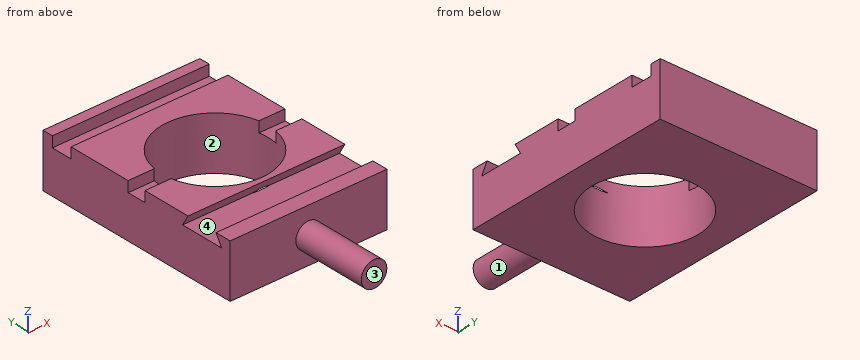
```python
from build123d import *

# Parameters (mm, degrees)
F1_W      = 73.6989242806
F1_H      = 100
F1_R      = 25
F2_DEPTH  = 100
F3_W      = 73.6989242806
F3_H      = 10
F4_DEPTH  = 5
F6_DEPTH  = 73.6989242806
F0_W      = 73.6989242806
F0_H      = 100
F7_DEPTH  = 75
F8_DEPTH  = 75
F9_R      = 6
F10_DEPTH = 35


with BuildPart() as f2:
    # F1 (on face) → F2 (new body)
    with BuildSketch(Plane.XY):
        Rectangle(F1_W, F1_H)
        Circle(F1_R, mode=Mode.SUBTRACT)
    extrude(amount=F2_DEPTH)

    # F3 (on face) → F4 (cut)
    with BuildSketch(Plane.XY.offset(100)):
        with BuildLine():
            Line((-24.5916652547, 4.5), (-36.8494621403, 4.5))
            Line((-36.8494621403, 4.5), (-36.8494621403, -4.5))
            Line((-36.8494621403, -4.5), (-24.5916652547, -4.5))
            ThreePointArc((-24.5916652547, -4.5), (-25, 0), (-24.5916652547, 4.5))
        make_face()
        with BuildLine():
            Line((36.8494621403, -4.5), (36.8494621403, 4.5))
            Line((36.8494621403, 4.5), (24.5916652547, 4.5))
            ThreePointArc((24.5916652547, 4.5), (24.8977070367, 2.2592441913), (25, 0))
            ThreePointArc((25, 0), (24.8977070367, -2.2592441913), (24.5916652547, -4.5))
            Line((24.5916652547, -4.5), (36.8494621403, -4.5))
        make_face()
        with Locations((0, 40)):
            Rectangle(F3_W, F3_H)
    extrude(amount=-F4_DEPTH, mode=Mode.SUBTRACT)

    # F5 (on face) → F6 (cut, through all)
    with BuildSketch(Plane(origin=(-36.8494621403, 0, 0), x_dir=(0, -1, 0), z_dir=(-1, 0, 0))):
        Polygon((42.5, 100), (27.5, 100), (24.6132486541, 95), (45.3867513459, 95), align=None)
    extrude(amount=-F6_DEPTH, mode=Mode.SUBTRACT)

    # F0 (on Top) → F7 (cut)
    with BuildSketch(Plane.XY):
        Rectangle(F0_W, F0_H)
    extrude(amount=-F7_DEPTH, mode=Mode.SUBTRACT)

    # F8 (cut): a face of the model
    f8_faces = [f2.faces().sort_by_distance(p)[0] for p in [
        (0, -48.7577628471, 0),
    ]]
    extrude(f8_faces, amount=-F8_DEPTH, mode=Mode.SUBTRACT)

    # F9 (on face) → F10 (join)
    with BuildSketch(Plane.XZ.offset(50)):
        with Locations((0, 87.5)):
            Circle(F9_R)
    extrude(amount=F10_DEPTH)


solid = f2.part
```
The listing builds one solid part. Answer for the finished solid, in the listing's coordinates (mm). Face numbers are marked on the shaded views. Round coordinates to 2 decimals unless told otherwise and drop trailing zeros. Write each loop counter-clockwise with the first axis right and the second up, starting at its lowest first coordinate (ties: lowest second). Pieces come first, ordered by that corner, then holes. Notation, with made-up numbers: (18, 14) -> (37, 14) arc R20 cw to (37, 49) -> close; hole circle Ø1 at (42.5, 46.5). An arc over 180 degrees is marked (long way). Answer as a JSON object with one key per item and string values. Group by question number.
Q1. Section A-A (y = 0) is taken. Write down the section's boundary in (x, z).
Q2. Each of these flat-tipped pins is pushed along its axis until it touches: pin 1 Ø10.5 at (x, y) = (3, -33.5) entering from +Z; pin 2 Ø10 at (x, z) = (19, 92.5) entering from -Y; pin 3 Ø8 at (y, z) = (-69, 84) entering from +X. Where does it stop, or does it pass through?
Q3. Determine the mould class of the marked faces 1, 2, 3 and 4 for opening direction Y: pulls with the +Y half, pulls with the -Y half, needs draft (parallel to the pull), parting line crosses it, or undercut.
Q4. Straight lines are drawn through the part: line 1 along X through (y, z) = (0, 87.25); line 2 along Y through (x, z) = (0, 82.25); line 3 along Y through (x, z) = (-4.5, 78.75). For each, find the intervals that lie inside material, in ascending order.
Q5. Section C-C (z = 87.5) is taken. Write down the section's boundary in (x, y), plus the area to 3 significant figures.
Q6. Section B-B (x = -21) is taken. Write down the section's boundary in (y, z), plus the area to 3 significant figures.
Q7. Section D-D (x = 0) is taken. Write down the section's boundary in (y, z).
Check values:
{
 "1": {"outline": "(-36.85, 75) -> (-25, 75) -> (-25, 95) -> (-36.85, 95) -> close; (25, 75) -> (36.85, 75) -> (36.85, 95) -> (25, 95) -> close"},
 "2": {"pin 1": "z = 95", "pin 2": "y = -50", "pin 3": "x = 6"},
 "3": {"face 1": "needs draft", "face 2": "undercut", "face 3": "pulls with the -Y half", "face 4": "undercut"},
 "4": {"line 1": "-36.85 to -25, 25 to 36.85", "line 2": "-85 to -25, 25 to 50", "line 3": "-50 to -24.59, 24.59 to 50"},
 "5": {"outline": "(-36.85, -50) -> (-6, -50) -> (-6, -85) -> (6, -85) -> (6, -50) -> (36.85, -50) -> (36.85, 50) -> (-36.85, 50) -> close; hole circle Ø50 at (0, 0)", "area": "5,830 mm^2"},
 "6": {"outline": "(-50, 75) -> (-13.56, 75) -> (-13.56, 100) -> (-27.5, 100) -> (-24.61, 95) -> (-45.39, 95) -> (-42.5, 100) -> (-50, 100) -> close; (13.56, 75) -> (50, 75) -> (50, 100) -> (45, 100) -> (45, 95) -> (35, 95) -> (35, 100) -> (13.56, 100) -> close", "area": "1,680 mm^2"},
 "7": {"outline": "(-85, 81.5) -> (-50, 81.5) -> (-50, 75) -> (-25, 75) -> (-25, 95) -> (-45.39, 95) -> (-42.5, 100) -> (-50, 100) -> (-50, 93.5) -> (-85, 93.5) -> close; (-27.5, 100) -> (-25, 95.67) -> (-25, 100) -> close; (25, 75) -> (50, 75) -> (50, 100) -> (45, 100) -> (45, 95) -> (35, 95) -> (35, 100) -> (25, 100) -> close"}
}
